```python
from build123d import *

# Parameters (mm, degrees)
CYLINDER001_R             = 2.5
CYLINDER001_DEPTH         = 4
CYLINDER_R                = 6.5
CYLINDER_DEPTH            = 25
BOX_W                     = 45
BOX_H                     = 50
BOX_DEPTH                 = 43
BOX001_W                  = 7
BOX001_H                  = 17
BOX001_DEPTH              = 10
FUSION001_PITCH_ANGLE     = -90
FUSION001_PLACEMENT_ANGLE = -180


with BuildPart() as obj1:
    # Cylinder001 → Cylinder001 (new body)
    with BuildSketch(Plane(origin=(10, 10, 43), x_dir=(1, 0, 0), z_dir=(0, 0, 1))):
        Circle(CYLINDER001_R)
    extrude(amount=CYLINDER001_DEPTH)


with BuildPart() as obj2:
    # Link001 base: copy of obj1
    add(obj1.part)


with BuildPart() as obj2_1:
    # Link001 placement: moved
    add(obj2.part.moved(Location((30, 0, 0))))


with BuildPart() as obj3:
    # Link base: copy of obj1
    add(obj1.part)


with BuildPart() as obj3_1:
    # Link placement: moved
    add(obj3.part.moved(Location((0, 30, 0))))


with BuildPart() as rotor:
    # Cylinder → Cylinder (new body)
    with BuildSketch(Plane(origin=(25, 25, 43), x_dir=(1, 0, 0), z_dir=(0, 0, 1))):
        Circle(CYLINDER_R)
    extrude(amount=CYLINDER_DEPTH)


with BuildPart() as base_motor:
    # Box → Box (new body)
    with BuildSketch(Plane.XY):
        with Locations((22.5, 25)):
            Rectangle(BOX_W, BOX_H)
    extrude(amount=BOX_DEPTH)


with BuildPart() as carcasa_motor:
    # Box001 → Box001 (new body)
    with BuildSketch(Plane(origin=(45, 16.5, 0), x_dir=(1, 0, 0), z_dir=(0, 0, 1))):
        with Locations((3.5, 8.5)):
            Rectangle(BOX001_W, BOX001_H)
    extrude(amount=BOX001_DEPTH)

    # Fusion: union Base Motor
    add(base_motor.part)


with BuildPart() as motor:
    # Link002 base: copy of obj1
    add(obj1.part)


with BuildPart() as motor_1:
    # Link002 placement: moved
    add(motor.part.moved(Location((30, 30, 0))))

    # Fusion001: union obj2, obj3, obj1, Rotor, Carcasa motor
    add(obj2_1.part)
    add(obj3_1.part)
    add(obj1.part)
    add(rotor.part)
    add(carcasa_motor.part)


with BuildPart() as motor_2:
    # Fusion001 pitch: moved
    add(motor_1.part.rotate(Axis((0, 0, 0), (0, 1, 0)), FUSION001_PITCH_ANGLE))


with BuildPart() as motor_3:
    # Fusion001 placement: moved
    add(motor_2.part.moved(Location((0, 25, 7))).rotate(Axis((0, 25, 7), (0, 0, 1)), FUSION001_PLACEMENT_ANGLE))


solid = motor_3.part
```
Here's how the part is built. I have some questions about the finished solid (model axes, mm). A direction names the side the tool comes from. Give positions to 0.01 mm unless a question says otherwise; leave off trailing zeros. Order: outer loops, then holes, each group sorted by start corner. A loop starts at its lowest first (then second) coordinate and runs counter-clockwise, first axis right, second up. Notation, with made-up numbers: (-17.75, 53) -> (37.25, 53) arc R23 ccw to (37.25, 66) -> close; hole circle Ø6 at (-18.75, -39). An arc over 180 degrees is marked (long way). Use CSV: the item, a comma, the result in double quotes. Start each with the question number.
Item 1: I'm going to push flat-ended pins straight in: P1, Ø7.5, axis at x = 6.5, z = 56.5, coming from the +Y side; P2, Ø3.5, axis at x = 7, z = 56, coming from the -Y side; P3, Ø4, axis at y = 14, z = 47, coming from the +X side. Where does each tip first touch, or does it pass through?
Item 2: Suppose I cut it at D-D (z = 17). List the corners of the cut face in (x, y) for me.
Item 3: Suppose I cut it at A-A (y = -15). List the corners of the cut face in (x, z) for me, and give its area (4 significant figures).
Item 4: Thinking about a two-plate mould opening in Z: for faces 1 (the cylindrical face through (55.325, -0.286, 25.506)), 2 (the flat face through (47, -15, 47)), 3 (the cylindrical face through (44.97, -14.04, 49.31)), 4 (the cylindrical face through (45, 14.9, 14.5)), which applies, pulls with the +Z half, pulls with the -Z half, needs draft (parallel to the pull), parting line crosses it, or undercut?
Item 5: If I drill on probe 1 along Z at (x, y) = (24, -18.5); probe 2 along X at (y, z) = (-13, 32); probe 3 along Y at (x, z) = (4.5, 54), over which ranges is the centre line in solid material (lowest first)? Write a range as [from, to].
Item 6: On a 3-axis mill with a long thin cutter (end or side, diameter ignored), from which of +Z, -Z, +X, -X, +Y, -Y can I reach the whole of each face in a straight line? I mean faces 5 (the flat face through (10, 0, 55)), 6 (the flat face through (5, -8.5, 55)), 7 (the flat face through (5, 8.5, 55)), 8 (the cylindrical face through (44.97, 15.96, 49.31)). Say none if no direction works.
Item 7: Suppose I cut it at B-B (z = 32). List the corners of the cut face in (x, y) for me.
Item 8: Suppose I cut it at C-C (x = 31.5). List the corners of the cut face in (y, z) for me, and give its area (3 significant figures).
Answer block:
1,P1,"stops at y = 8.5"
1,P2,"stops at y = -8.5"
1,P3,"stops at x = 47"
2,outline,"(0, -25) -> (43, -25) -> (43, -17.5) -> (47, -17.5) -> (47, -12.5) -> (43, -12.5) -> (43, 12.5) -> (47, 12.5) -> (47, 17.5) -> (43, 17.5) -> (43, 25) -> (0, 25) -> close"
3,outline,"(0, 7) -> (43, 7) -> (43, 14.5) -> (47, 14.5) -> (47, 19.5) -> (43, 19.5) -> (43, 44.5) -> (47, 44.5) -> (47, 49.5) -> (43, 49.5) -> (43, 52) -> (0, 52) -> close"
3,area,"1,975 mm^2"
4,face 1,"parting line crosses it"
4,face 2,"needs draft"
4,face 3,"undercut"
4,face 4,"undercut"
5,probe 1,"z = [7, 52]"
5,probe 2,"x = [0, 43]"
5,probe 3,"y = [-8.5, 8.5]"
6,face 5,"+Z, +X, +Y, -Y"
6,face 6,"+Z, +X, -X, -Y"
6,face 7,"+Z, +X, -X, +Y"
6,face 8,"+X"
7,outline,"(0, -25) -> (43, -25) -> (43, -6.5) -> (68, -6.5) -> (68, 6.5) -> (43, 6.5) -> (43, 25) -> (0, 25) -> close"
8,outline,"(-25, 7) -> (25, 7) -> (25, 52) -> (-25, 52) -> close"
8,area,"2,250 mm^2"
